from build123d import *

# Parameters (mm, degrees)
SKETCH1_W                      = 280
SKETCH1_H                      = 100
BOSS_EXTRUDE1_DEPTH            = 1
SKETCH2_W                      = 50
SKETCH2_H                      = 50
CUT_EXTRUDE3_DEPTH             = 149.664050799
CUT_EXTRUDE4_DEPTH             = 149.664050799
EDGE_FLANGE1_STRIP_W           = 6
EDGE_FLANGE1_STRIP_H           = 1
EDGE_FLANGE1_STRIP_CUT_DEPTH   = 100
EDGE_FLANGE1_STRIP_2_W         = 6
EDGE_FLANGE1_STRIP_2_H         = 1
EDGE_FLANGE1_STRIP_CUT_2_DEPTH = 100
EDGE_FLANGE1_DEPTH             = 100
EDGE_FLANGE1_BEND_DEPTH        = 100
EDGE_FLANGE2_STRIP_W           = 6
EDGE_FLANGE2_STRIP_H           = 1
EDGE_FLANGE2_STRIP_CUT_DEPTH   = 100
EDGE_FLANGE2_STRIP_2_W         = 6
EDGE_FLANGE2_STRIP_2_H         = 1
EDGE_FLANGE2_STRIP_CUT_2_DEPTH = 100
EDGE_FLANGE2_DEPTH             = 100
EDGE_FLANGE2_BEND_DEPTH        = 100
CUT_EXTRUDE5_DEPTH             = 168.755774863


# Sheet-metal steps are written as plain solids
with BuildPart() as part:
    # Sketch1 → Boss-Extrude1 (new body)
    with BuildSketch(Plane.YZ):
        Rectangle(SKETCH1_W, SKETCH1_H)
    extrude(amount=BOSS_EXTRUDE1_DEPTH)

    # Sketch2 → Cut-Extrude3 (cut, through all)
    with BuildSketch(Plane.YZ.offset(1)):
        with Locations((-55, 25)):
            Rectangle(SKETCH2_W, SKETCH2_H)
        with Locations((55, 25)):
            Rectangle(SKETCH2_W, SKETCH2_H)
    extrude(amount=-CUT_EXTRUDE3_DEPTH, mode=Mode.SUBTRACT)

    # Sketch3 → Cut-Extrude4 (cut, through all)
    with BuildSketch(Plane.YZ.offset(1)):
        with BuildLine():
            Line((-16.6, 40), (-16.6, 44))
            ThreePointArc((-16.6, 44), (-15, 45.6), (-13.4, 44))
            Line((-13.4, 44), (-13.4, 40))
            ThreePointArc((-13.4, 40), (-15, 38.4), (-16.6, 40))
        make_face()
        with BuildLine():
            Line((13.4, 40), (13.4, 44))
            ThreePointArc((13.4, 44), (15, 45.6), (16.6, 44))
            Line((16.6, 44), (16.6, 40))
            ThreePointArc((16.6, 40), (15, 38.4), (13.4, 40))
        make_face()
        with BuildLine():
            Line((13.4, 10), (13.4, 14))
            ThreePointArc((13.4, 14), (15, 15.6), (16.6, 14))
            Line((16.6, 14), (16.6, 10))
            ThreePointArc((16.6, 10), (15, 8.4), (13.4, 10))
        make_face()
        with BuildLine():
            Line((-16.6, 10), (-16.6, 14))
            ThreePointArc((-16.6, 14), (-15, 15.6), (-13.4, 14))
            Line((-13.4, 14), (-13.4, 10))
            ThreePointArc((-13.4, 10), (-15, 8.4), (-16.6, 10))
        make_face()
    extrude(amount=-CUT_EXTRUDE4_DEPTH, mode=Mode.SUBTRACT)

    # Edge-Flange1 strip (across the edge) → Edge-Flange1 strip cut (cut)
    with BuildSketch(Plane(origin=(1, 140, -50), x_dir=(0, -1, 0), z_dir=(0, 0, 1))):
        with Locations((-1, -0.5)):
            Rectangle(EDGE_FLANGE1_STRIP_W, EDGE_FLANGE1_STRIP_H)
    extrude(amount=EDGE_FLANGE1_STRIP_CUT_DEPTH, mode=Mode.SUBTRACT)

    # Edge-Flange1 strip 2 (across the edge) → Edge-Flange1 strip cut 2 (cut)
    with BuildSketch(Plane(origin=(1, -140, 50), x_dir=(0, 1, 0), z_dir=(0, 0, -1))):
        with Locations((-1, -0.5)):
            Rectangle(EDGE_FLANGE1_STRIP_2_W, EDGE_FLANGE1_STRIP_2_H)
    extrude(amount=EDGE_FLANGE1_STRIP_CUT_2_DEPTH, mode=Mode.SUBTRACT)

    # Edge-Flange1 section (across the edge) → Edge-Flange1 (add)
    with BuildSketch(Plane(origin=(1, 140, -50), x_dir=(0, -1, 0), z_dir=(0, 0, 1))):
        with BuildLine():
            Line((0, 1), (0, 18))
            Line((0, 18), (1, 18))
            Line((1, 18), (1, 1))
            ThreePointArc((1, 1), (1.292893219, 0.292893219), (2, 0))
            Line((2, 0), (2, -1))
            ThreePointArc((2, -1), (0.585786438, -0.414213562), (0, 1))
        make_face()
    extrude(amount=EDGE_FLANGE1_DEPTH)

    # Edge-Flange1 section 2 (across the edge) → Edge-Flange1 bend (add)
    with BuildSketch(Plane(origin=(1, -140, 50), x_dir=(0, 1, 0), z_dir=(0, 0, -1))):
        with BuildLine():
            Line((0, 1), (0, 18))
            Line((0, 18), (1, 18))
            Line((1, 18), (1, 1))
            ThreePointArc((1, 1), (1.292893219, 0.292893219), (2, 0))
            Line((2, 0), (2, -1))
            ThreePointArc((2, -1), (0.585786438, -0.414213562), (0, 1))
        make_face()
    extrude(amount=EDGE_FLANGE1_BEND_DEPTH)

    # Edge-Flange2 strip (across the edge) → Edge-Flange2 strip cut (cut)
    with BuildSketch(Plane(origin=(19, 140, 50), x_dir=(-1, 0, 0), z_dir=(0, 0, -1))):
        with Locations((-1, -0.5)):
            Rectangle(EDGE_FLANGE2_STRIP_W, EDGE_FLANGE2_STRIP_H)
    extrude(amount=EDGE_FLANGE2_STRIP_CUT_DEPTH, mode=Mode.SUBTRACT)

    # Edge-Flange2 strip 2 (across the edge) → Edge-Flange2 strip cut 2 (cut)
    with BuildSketch(Plane(origin=(19, -140, -50), x_dir=(-1, 0, 0), z_dir=(0, 0, 1))):
        with Locations((-1, -0.5)):
            Rectangle(EDGE_FLANGE2_STRIP_2_W, EDGE_FLANGE2_STRIP_2_H)
    extrude(amount=EDGE_FLANGE2_STRIP_CUT_2_DEPTH, mode=Mode.SUBTRACT)

    # Edge-Flange2 section (across the edge) → Edge-Flange2 (add)
    with BuildSketch(Plane(origin=(19, 140, 50), x_dir=(-1, 0, 0), z_dir=(0, 0, -1))):
        with BuildLine():
            Line((0, 1), (0, 19))
            Line((0, 19), (1, 19))
            Line((1, 19), (1, 1))
            ThreePointArc((1, 1), (1.292893219, 0.292893219), (2, 0))
            Line((2, 0), (2, -1))
            ThreePointArc((2, -1), (0.585786438, -0.414213562), (0, 1))
        make_face()
    extrude(amount=EDGE_FLANGE2_DEPTH)

    # Edge-Flange2 section 2 (across the edge) → Edge-Flange2 bend (add)
    with BuildSketch(Plane(origin=(19, -140, -50), x_dir=(-1, 0, 0), z_dir=(0, 0, 1))):
        with BuildLine():
            Line((0, 1), (0, 19))
            Line((0, 19), (1, 19))
            Line((1, 19), (1, 1))
            ThreePointArc((1, 1), (1.292893219, 0.292893219), (2, 0))
            Line((2, 0), (2, -1))
            ThreePointArc((2, -1), (0.585786438, -0.414213562), (0, 1))
        make_face()
    extrude(amount=EDGE_FLANGE2_BEND_DEPTH)

    # Sketch26 → Cut-Extrude5 (cut, through all)
    with BuildSketch(Plane.YZ.offset(19)):
        Polygon((-149.792397295, 45.041451884), (-153.292397295, 43.020725942), (-153.292397295, 38.979274058), (-149.792397295, 36.958548116), (-146.292397295, 38.979274058), (-146.292397295, 43.020725942), align=None)
        Polygon((-149.792397295, -36.958548116), (-153.292397295, -38.979274058), (-153.292397295, -43.020725942), (-149.792397295, -45.041451884), (-146.292397295, -43.020725942), (-146.292397295, -38.979274058), align=None)
        Polygon((147.707602705, -43.020725942), (151.207602705, -45.041451884), (154.707602705, -43.020725942), (154.707602705, -38.979274058), (151.207602705, -36.958548116), (147.707602705, -38.979274058), align=None)
        Polygon((147.707602705, 38.979274058), (151.207602705, 36.958548116), (154.707602705, 38.979274058), (154.707602705, 43.020725942), (151.207602705, 45.041451884), (147.707602705, 43.020725942), align=None)
    extrude(amount=-CUT_EXTRUDE5_DEPTH, mode=Mode.SUBTRACT)


solid = part.part
CAD build for the part. Positions are in the model's coordinates, mm. A direction names the side the tool comes from. Coordinates: 2 decimals unless noted, no trailing zeros. Order: outer loops, then holes, each group sorted by start corner. A loop starts at its lowest first (then second) coordinate and runs counter-clockwise, first axis right, second up. Notation, with made-up numbers: (68, 21) -> (101, 21) arc R31 cw to (101, 59) -> close; hole circle Ø9 at (54.5, 31.25). An arc over 180 degrees is marked (long way). Answer in a Markdown table with one row per item.
1) Mould opens along Y. For faces 1 (the face through (18, -150, -1)), 2 (the face through (1, -2, 1)), 3 (the face through (9, 140, -1)), 4 (the face through (10, 139, -1)) say: pulls with the +Y half, pulls with the -Y half, needs draft (parallel to the pull), parting line crosses it, or undercut.
Check values:
| item | result |
|---|---|
| face 1 | needs draft |
| face 2 | undercut |
| face 3 | pulls with the +Y half |
| face 4 | undercut |
2) Band-saw the part on C-C (y = 2.5). List the corners of the cut face in (x, z).
Check values:
| item | result |
|---|---|
| outline | (0, -50) -> (1, -50) -> (1, 50) -> (0, 50) -> close |
3) Which spindle directions (+Z, -Z, +X, -X, +Y, -Y) get a long thin tool onto all of the face, cutting with end or side? Do faces 5 (the face through (10, -139, 1)), 6 (the face through (0, -2, 1)), 7 (the face through (9, -140, 1)), 8 (the face through (19, 150, 1)), 9 (the face through (18, 150, 1)). Say none if no direction does.
Check values:
| item | result |
|---|---|
| face 5 | +Z, -Z, +X |
| face 6 | +Z, -Z, -X, +Y, -Y |
| face 7 | +Z, -Z, -X, -Y |
| face 8 | +Z, -Z, +X, +Y, -Y |
| face 9 | +Z, -Z, -X, +Y |
4) Drill centre lines: line 1 (Y direction, x = 13.5, z = 21.5); line 2 (X direction, y = -13, z = 40.5); line 3 (X direction, y = 142, z = 45). Where is each one in solid material? Low to high.
Check values:
| item | result |
|---|---|
| line 1 | -140 to -139, 139 to 140 |
| line 2 | 0 to 1 |
| line 3 | 18 to 19 |
5) Flat gauge pins, fed straight in: P1, Ø1.1, axis at x = 0.5, z = 11.5, coming from the +Y side; P2, Ø8, axis at x = 3.5, z = 36, coming from the -Y side; P3, Ø20, axis at y = 152, z = -10, coming from the -X side. Where does each tip first touch, or does it go through?
Check values:
| item | result |
|---|---|
| P1 | y = 139.76 |
| P2 | y = -140 |
| P3 | x = 18 |
6) Band-saw the part on D-D (y = 56.5). List the corners of the cut face in (x, z).
Check values:
| item | result |
|---|---|
| outline | (0, -50) -> (1, -50) -> (1, 0) -> (0, 0) -> close |
7) Band-saw the part on B-B (x = 6). List the corners of the cut face in (y, z).
Check values:
| item | result |
|---|---|
| outline | (-140, -50) -> (-139, -50) -> (-139, 50) -> (-140, 50) -> close; (139, -50) -> (140, -50) -> (140, 50) -> (139, 50) -> close |
8) Band-saw the part on A-A (z = 28). List the corners of the cut face in (x, y), and give its area (3 significant figures).
Check values:
| item | result |
|---|---|
| outline | (0, -138) arc R2 ccw to (2, -140) -> (17, -140) arc R1 cw to (18, -141) -> (18, -159) -> (19, -159) -> (19, -141) arc R2 ccw to (17, -139) -> (2, -139) arc R1 cw to (1, -138) -> (1, -80) -> (0, -80) -> close; (0, -30) -> (1, -30) -> (1, 30) -> (0, 30) -> close; (0, 80) -> (1, 80) -> (1, 138) arc R1 cw to (2, 139) -> (17, 139) arc R2 ccw to (19, 141) -> (19, 159) -> (18, 159) -> (18, 141) arc R1 cw to (17, 140) -> (2, 140) arc R2 ccw to (0, 138) -> close |
| area | 251 mm2 |
